Part model, mm, in its own coordinate system. Face numbers are marked on the shaded views. A direction names the side the tool comes from. Give positions to 0.01 mm unless a question says otherwise; leave off trailing zeros. Order: outer loops, then holes, each group sorted by start corner. A loop starts at its lowest first (then second) coordinate and runs counter-clockwise, first axis right, second up.
1. Probe line 1 (Z direction, x = 4, y = 2.75); line 2 (Z direction, x = 0, y = 0); line 3 (X direction, y = -4.75, z = 10). List the from-to ranges inside material, lowest first.
2. Slice it at A-A on z = 0. List the corners of the cut face in (x, y) (3 decimals).
3. Which spindle directions (+Z, -Z, +X, -X, +Y, -Y) get a long thin tool onto all of the face, cutting with end or side? Do the marked faces 1, 2 and 3. Say none if no direction does.
4. Drop flat-ended pins along their axis: pin 1 Ø4.5 at (y, z) = (7.5, -1) entering from -X; pin 2 Ø6.5 at (y, z) = (-0.5, -12) entering from +X; pin 3 Ø1 at (x, z) = (-21.5, 18.5) entering from +Y. Give the stop position or say it passes through.
5. Slice it at D-D on y = -1.25. List the corners of the cut face in (x, z).
6. Slice it at C-C on x = 0. List the corners of the cut face in (y, z), and give its area (3 significant figures).
7. Slice it at B-B on y = 12.75. List the corners of the cut face in (x, z) (3 decimals), and give its area (3 significant figures).
8. Mould opens along X. For the marked faces 4 and 5 say: +X half, -X half, draft (parallel to the pull), parting line (faces both ways), or undercut.
from build123d import *

# Parameters (mm, degrees)
BOSS_EXTRUDE1_DEPTH      = 4
BOSS_EXTRUDE1_DEPTH_BACK = 4
SKETCH4_R                = 5
BOSS_EXTRUDE2_DEPTH      = 10
CUT_EXTRUDE1_DEPTH       = 9


with BuildPart() as part:
    # Sketch2 → Revolve1 (revolve)
    with BuildSketch(Plane.XY, mode=Mode.PRIVATE) as revolve1_sk:
        with BuildLine():
            Line((-19, -4.5), (-19, 4.5))
            Line((-19, 4.5), (-23, 7))
            Line((-23, 7), (-30, 7))
            ThreePointArc((-30, 7), (-32.5, 0), (-30, -7))
            Line((-30, -7), (-23, -7))
            Line((-23, -7), (-19, -4.5))
        make_face()
    revolve(revolve1_sk.sketch.rotate(Axis((0, -7, 0), (0, 1, 0)), 180), axis=Axis((0, -7, 0), (0, 1, 0)))

    # Sketch3 → Boss-Extrude1 (add, two sides: drawn at the far end of the back side and taken through both)
    with BuildSketch(Plane(origin=(0, 0, 0), x_dir=(1, 0, 0), z_dir=(0, 1, 0)).offset(-BOSS_EXTRUDE1_DEPTH_BACK)):
        with BuildLine():
            Line((9, 3), (25, 3))
            Line((25, 3), (25, -3))
            Line((25, -3), (9, -3))
            ThreePointArc((9, -3), (4.757359313, -4.757359313), (3, -9))
            Line((3, -9), (3, -25))
            Line((3, -25), (-3, -25))
            Line((-3, -25), (-3, -9))
            ThreePointArc((-3, -9), (-4.757359313, -4.757359313), (-9, -3))
            Line((-9, -3), (-25, -3))
            Line((-25, -3), (-25, 3))
            Line((-25, 3), (-9, 3))
            ThreePointArc((-9, 3), (-4.757359313, 4.757359313), (-3, 9))
            Line((-3, 9), (-3, 25))
            Line((-3, 25), (3, 25))
            Line((3, 25), (3, 9))
            ThreePointArc((3, 9), (4.757359313, 4.757359313), (9, 3))
        make_face()
    extrude(amount=BOSS_EXTRUDE1_DEPTH + BOSS_EXTRUDE1_DEPTH_BACK)

    # Sketch4 → Boss-Extrude2 (add)
    with BuildSketch(Plane(origin=(0, 4, 0), x_dir=(1, 0, 0), z_dir=(0, 1, 0))):
        with Locations(Location((0, 0, 0), (0, 0, 180))):
            Circle(SKETCH4_R)
    extrude(amount=BOSS_EXTRUDE2_DEPTH)

    # Sketch5 → Cut-Extrude1 (cut)
    with BuildSketch(Plane(origin=(0, 14, 0), x_dir=(1, 0, 0), z_dir=(0, 1, 0))):
        with BuildLine():
            Line((-1.885, -2.017231601), (-1.885, 2.002198265))
            ThreePointArc((-1.885, 2.002198265), (0.011383629, 2.727171226), (1.885, 1.945238778))
            Line((1.885, 1.945238778), (1.885, -1.960272114))
            ThreePointArc((1.885, -1.960272114), (0.011383629, -2.742204562), (-1.885, -2.017231601))
        make_face()
    extrude(amount=-CUT_EXTRUDE1_DEPTH, mode=Mode.SUBTRACT)


solid = part.part
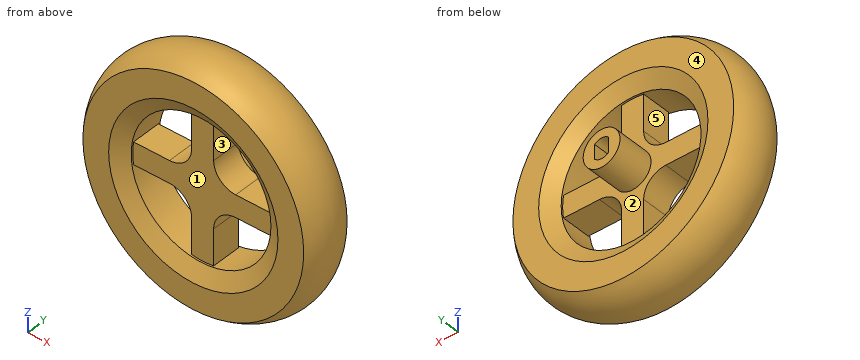
Data:
1. line 1: z = -31.9 to -18.57, -5.68 to 5.68, 18.57 to 31.9
1. line 2: z = -32.5 to 32.5
1. line 3: x = -29.79 to -16.62, 16.62 to 29.79
2. outline: (-30, -7) - (-23, -7) - (-19, -4.5) - (-19, -4) - (19, -4) - (19, -4.5) - (23, -7) - (30, -7) arc R11.05 ccw to (30, 7) - (23, 7) - (19, 4.5) - (19, 4) - (5, 4) - (5, 14) - (1.885, 14) - (1.885, 5) - (-1.885, 5) - (-1.885, 14) - (-5, 14) - (-5, 4) - (-19, 4) - (-19, 4.5) - (-23, 7) - (-30, 7) arc R11.05 ccw to start
3. face 1: -Y
3. face 2: +Y
3. face 3: +Y, -Y
4. pin 1: stops at x = -31.16
4. pin 2: stops at x = 31.29
4. pin 3: stops at y = 7
5. outline: circle Ø64.86 at (0, 0); hole (-18.76, -3) arc R19 ccw to (-3, -18.76) - (-3, -9) arc R6 ccw to (-9, -3) - close; hole (-18.76, 3) - (-9, 3) arc R6 ccw to (-3, 9) - (-3, 18.76) arc R19 ccw to start; hole (3, -18.76) arc R19 ccw to (18.76, -3) - (9, -3) arc R6 ccw to (3, -9) - close; hole (3, 9) arc R6 ccw to (9, 3) - (18.76, 3) arc R19 ccw to (3, 18.76) - close
6. outline: (-7, -30) arc R11.05 ccw to (7, -30) - (7, -23) - (4.5, -19) - (4, -19) - (4, -5) - (14, -5) - (14, -2.73) - (5, -2.73) - (5, 2.74) - (14, 2.74) - (14, 5) - (4, 5) - (4, 19) - (4.5, 19) - (7, 23) - (7, 30) arc R11.05 ccw to (-7, 30) - (-7, 23) - (-4.5, 19) - (-4, 19) - (-4, -19) - (-4.5, -19) - (-7, -23) - close
6. area: 691 mm2
7. outline: circle Ø10 at (0, 0); hole (-1.885, -2.002) arc R2.735 ccw to (1.885, -1.945) - (1.885, 1.96) arc R2.735 ccw to (-1.885, 2.017) - close
7. area: 59.7 mm2
8. face 4: draft
8. face 5: undercut
